Geometry check sheet. Reference: the model listing, model coordinates, mm. A direction names the side the tool comes from. Give positions to 0.01 mm unless a question says otherwise; leave off trailing zeros. Write each loop counter-clockwise with the first axis right and the second up, starting at its lowest first coordinate (ties: lowest second). Pieces come first, ordered by that corner, then holes.
(1) Mould release check, pull along X, two halves, no side actions. Record for faces 1 (the flat face through (-2.1, 2, -153)), 2 (the flat face through (3, 0, -148)), 3 (the flat face through (-4, 2, -148)): +X half, -X half, draft (parallel to the pull), parting line (faces both ways), or undercut.
(2) Thickness scan on line 1 along Z through (x, y) = (0, 3.8); line 2 along X through (y, z) = (3.7, -221); line 3 along Z through (x, y) = (-1, 2.75). Record the ranges inside material, lowest first.
(3) Cross-section at C-C (y = 4). Record the boundary of the cut face in (x, z), and give its area (3 significant figures).
(4) Tool access check on faces 4 (the flat face through (3, 5, -148)), 5 (the flat face through (2.1, 2, -157)). Record the directions out of +Z, -Z, +X, -X, +Y, -Y that give a thin tool (end or side, any length) a straight path to the whole face; none if there is none.
(5) Cross-section at B-B (z = -232). Record the boundary of the cut face in (x, y), and give its area (3 significant figures).
(6) Cross-section at A-A (x = 0). Record the boundary of the cut face in (y, z).
Autodesk Inventor part; units mm, degrees
ref_plane "XZ Plane" through (0, 0, 0) normal (0, 1, 0) x (-1, 0, 0)
sketch "Sketch1" plane through (0, 0, 0) normal (0, 1, 0) x (-1, 0, 0)
  line L0 (0, 0) -> (0, -300) construction
  line L1 (4, 0) -> (4, -300)
  line L2 (-4, -300) -> (-4, 0)
  arc A0 (4, 0) -> (-4, 0) centre (0, 0) ccw
  arc A1 (-4, -300) -> (4, -300) centre (0, -300) ccw
  circle A2 centre (0, 0) radius 2.1
  line L3 (0, -10) -> (0, -300) construction
  line L4 (2.1, -10) -> (2.1, -300)
  line L5 (-2.1, -300) -> (-2.1, -10)
  arc A3 (2.1, -10) -> (-2.1, -10) centre (0, -10) ccw
  arc A4 (-2.1, -300) -> (2.1, -300) centre (0, -300) ccw
  point P0 (0, -150)
  point P1 (0, -155)
  dimension "d0" = 8
  dimension "d1" = 300
  dimension "d2" = 4.2
  dimension "d3" = 4.2
  dimension "d4" = 10
extrude "Extrusion1" add sketch "Sketch1" along normal blind 5
Reply:
1. face 1: undercut
1. face 2: draft
1. face 3: -X half
2. line 1: z = -304 to -302.1, -7.9 to -2.1, 2.1 to 4
2. line 2: x = -4 to -2.1, 2.1 to 4
2. line 3: z = -303.87 to -301.85, -8.15 to -1.85, 1.85 to 3.87
3. outline: (-4, -300) arc R4 ccw to (4, -300) - (4, 0) arc R4 ccw to (-4, 0) - close; hole (-2.1, -300) arc R2.1 ccw to (2.1, -300) - (2.1, -10) arc R2.1 ccw to (-2.1, -10) - close; hole circle Ø4.2 at (0, 0)
3. area: 1,200 mm2
4. face 4: +Z, -Z, +X, -X, +Y
4. face 5: +Y, -Y
5. outline: (-4, 0) - (-2.1, 0) - (-2.1, 5) - (-4, 5) - close; (2.1, 0) - (4, 0) - (4, 5) - (2.1, 5) - close
5. area: 19.0 mm2
6. outline: (0, -304) - (5, -304) - (5, -302.1) - (0, -302.1) - close; (0, -7.9) - (5, -7.9) - (5, -2.1) - (0, -2.1) - close; (0, 2.1) - (5, 2.1) - (5, 4) - (0, 4) - close
